Geometry: final body of the model. Coordinates: model frame, mm. Face numbers are marked on the shaded views. A direction names the side the tool comes from. Give positions to 0.01 mm unless a question says otherwise; leave off trailing zeros. Write each loop counter-clockwise with the first axis right and the second up, starting at its lowest first coordinate (ties: lowest second). Pieces come first, ordered by that corner, then holes.
from build123d import *

# Parameters (mm, degrees)
SALIENTE_EXTRUIR1_DEPTH      = 45
SALIENTE_EXTRUIR2_DEPTH      = 3
SALIENTE_EXTRUIR3_REACH      = 75.192
SALIENTE_EXTRUIR3_END_RADIUS = 33
CROQUIS3_R                   = 6
SALIENTE_EXTRUIR4_START      = 5
CROQUIS4_R                   = 6
SALIENTE_EXTRUIR4_DEPTH      = 5
CROQUIS5_R                   = 3
CORTAR_EXTRUIR1_DEPTH        = 12


with BuildPart() as part:
    # Croquis1 → Saliente-Extruir1 (new body)
    with BuildSketch(Plane(origin=(0, 0, 0), x_dir=(1, 0, 0), z_dir=(0, 1, 0))):
        with BuildLine():
            Line((2.952769471, -3), (50.275773024, -3))
            ThreePointArc((50.275773024, -3), (52.944271247, 10), (50.275773024, 23))
            Line((50.275773024, 23), (2.952769471, 23))
            ThreePointArc((2.952769471, 23), (0.284271247, 10), (2.952769471, -3))
        make_face()
        with BuildLine():
            Line((5, 0), (48.228542495, 0))
            ThreePointArc((48.228542495, 0), (49.944271247, 10), (48.228542495, 20))
            Line((48.228542495, 20), (5, 20))
            ThreePointArc((5, 20), (3.284271247, 10), (5, 0))
        make_face(mode=Mode.SUBTRACT)
    extrude(amount=SALIENTE_EXTRUIR1_DEPTH)

    # Croquis2 → Saliente-Extruir2 (add)
    with BuildSketch(Plane.XZ):
        with BuildLine():
            Line((2.952769471, 3), (50.275773024, 3))
            ThreePointArc((50.275773024, 3), (52.944271247, -10), (50.275773024, -23))
            Line((50.275773024, -23), (2.952769471, -23))
            ThreePointArc((2.952769471, -23), (0.284271247, -10), (2.952769471, 3))
        make_face()
        with BuildLine():
            Line((15.114271247, -20), (38.114271247, -20))
            ThreePointArc((38.114271247, -20), (39.409874114, -10), (38.114271247, 0))
            Line((38.114271247, 0), (15.114271247, 0))
            ThreePointArc((15.114271247, 0), (13.398542495, -10), (15.114271247, -20))
        make_face(mode=Mode.SUBTRACT)
    extrude(amount=-SALIENTE_EXTRUIR2_DEPTH)

    # Saliente-Extruir3: up to this cylinder (the profile starts outside it)
    saliente_extruir3_end = Plane(origin=(33.284271247, 22.52988, -10), z_dir=(0, -1, 0)) * Cylinder(SALIENTE_EXTRUIR3_END_RADIUS, 217.384, mode=Mode.PRIVATE)
    # Croquis3 → Saliente-Extruir3 (add, up to the surface)
    with BuildSketch(Plane(origin=(0, 0, 0), x_dir=(0, 0, -1), z_dir=(1, 0, 0)), mode=Mode.PRIVATE) as saliente_extruir3_sk1:
        with Locations(Location((10, 22.52988005, 0), (0, 0, 180))):
            Circle(CROQUIS3_R)
    saliente_extruir3_tool1 = extrude(saliente_extruir3_sk1.sketch, amount=SALIENTE_EXTRUIR3_REACH, mode=Mode.PRIVATE) - saliente_extruir3_end
    add(saliente_extruir3_tool1.solids().sort_by_distance((0, 22.52988, -10))[0])

    # Croquis4 → Saliente-Extruir4 (add)
    with BuildSketch(Plane.ZY.offset(SALIENTE_EXTRUIR4_START)):
        with Locations((-10, 22.52988005)):
            Circle(CROQUIS4_R)
    extrude(amount=-SALIENTE_EXTRUIR4_DEPTH)

    # Croquis5 → Cortar-Extruir1 (cut)
    with BuildSketch(Plane.ZY.offset(5)):
        with Locations((-10, 22.52988005)):
            Circle(CROQUIS5_R)
    extrude(amount=-CORTAR_EXTRUIR1_DEPTH, mode=Mode.SUBTRACT)


solid = part.part
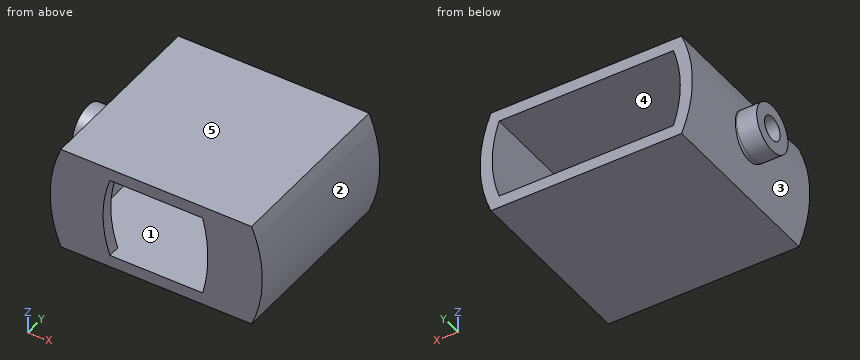
Q1. Pull-direction query (X, two-part tool) for the marked faces 1, 2 and 3; classes: released by +X, released by -X, zero draft, split by the parting line, or undercut.
Filled sheet:
face 1: undercut
face 2: released by +X
face 3: released by -X
Q2. Section B-B on x = 33. Output: boundary loops of the cut face in (y, z), plus the area to 3 significant figures.
Filled sheet:
outline: (0, -23) - (45, -23) - (45, -20) - (0, -20) - close; (0, 0) - (45, 0) - (45, 3) - (0, 3) - close
area: 270 mm2
Q3. Section A-A on z = -10. Output: boundary loops of the cut face in (x, y), plus the area to 3 significant figures.
Filled sheet:
outline: (-5, 16.53) - (0.28, 16.53) - (0.28, 0) - (13.4, 0) - (13.4, 3) - (3.28, 3) - (3.28, 19.53) - (-5, 19.53) - close; (-5, 25.53) - (3.28, 25.53) - (3.28, 45) - (0.28, 45) - (0.28, 28.53) - (-5, 28.53) - close; (39.41, 0) - (52.94, 0) - (52.94, 45) - (49.94, 45) - (49.94, 3) - (39.41, 3) - close
area: 346 mm2
Q4. Ray query, line 1 along Y through (x, z) = (1, -10); line 2 along Z through (x, y) = (42, 41.5); line 3 along Y through (x, z) = (0.25, -10). Return the intervals inside material, ascending.
Filled sheet:
line 1: y = 0 to 19.53, 25.53 to 45
line 2: z = -23 to -20, 0 to 3
line 3: y = 16.53 to 19.53, 25.53 to 28.53
Q5. Section C-C on y = 5.5. Output: boundary loops of the cut face in (x, z).
Filled sheet:
outline: (2.95, -23) - (50.28, -23) arc R33 ccw to (50.28, 3) - (2.95, 3) arc R33 ccw to start; hole (5, -20) - (48.23, -20) arc R30 ccw to (48.23, 0) - (5, 0) arc R30 ccw to start
Q6. Access query for the marked faces 4 and 5. Directions: +Z, -Z, +X, -X, +Y, -Y. A direction counts if a zero-diameter tool reaches every point of the face in a straight line with its end or side. Return the directions, or none.
Filled sheet:
face 4: +Y
face 5: +Z, +X, -X, +Y, -Y
Q7. Pin query (flat end, axial travel): P1, Ø8, axis at y = 6, z = -20, coming from the +X side; P2, Ø1, axis at x = 19, z = -19, coming from the -Y side (1 decimal); P3, Ø3, axis at x = 45, z = -19, coming from the -Y side; P4, Ø6, axis at x = 10.5, z = -7, coming from the +Y side. Return the tip coordinate at first contact, or that it passes through.
Filled sheet:
P1: stops at x = 52.39
P2: passes through
P3: stops at y = 0
P4: stops at y = 3
Q8. Section D-D on z = -19. Output: boundary loops of the cut face in (x, y), plus the area to 3 significant figures.
Filled sheet:
outline: (1.54, 0) - (14.78, 0) - (14.78, 3) - (4.67, 3) - (4.67, 45) - (1.54, 45) - close; (38.36, 0) - (51.69, 0) - (51.69, 45) - (48.56, 45) - (48.56, 3) - (38.36, 3) - close
area: 343 mm2
